```python
from build123d import *

# Parameters (mm, degrees)
BOSS_EXTRUDE1_DEPTH = 5.07492
SKETCH5_W           = 44.45
SKETCH5_H           = 127
BOSS_EXTRUDE2_DEPTH = 5.07492
SKETCH6_R           = 22.225
BOSS_EXTRUDE3_DEPTH = 5.07492
SKETCH2_3_R         = 6.35
CUT_EXTRUDE2_DEPTH  = 5.588
SKETCH8_W           = 2.728150378
SKETCH8_H           = 119.38
BOSS_EXTRUDE4_DEPTH = 5.07492
SKETCH9_R           = 3
CUT_EXTRUDE3_DEPTH  = 400.05
SKETCH10_R          = 2.54
SKETCH10_R_2        = 3.175
CUT_EXTRUDE4_DEPTH  = 6.35


with BuildPart() as part:
    # Sketch2 → Boss-Extrude1 (new body)
    with BuildSketch(Plane.XY):
        with BuildLine():
            Line((-143.383, -31.75), (-127.127, -31.75))
            ThreePointArc((-127.127, -31.75), (-123.317, -30.48), (-119.507, -31.75))
            Line((-119.507, -31.75), (119.253, -31.75))
            ThreePointArc((119.253, -31.75), (123.063, -30.48), (126.873, -31.75))
            Line((126.873, -31.75), (143.383, -31.75))
            Line((143.383, -31.75), (143.383, 95.25))
            Line((143.383, 95.25), (-143.383, 95.25))
            Line((-143.383, 95.25), (-143.383, -31.75))
        make_face()
    extrude(amount=-BOSS_EXTRUDE1_DEPTH)

    # Sketch5 → Boss-Extrude2 (add)
    with BuildSketch(Plane(origin=(0, 0, -5.07492), x_dir=(-1, 0, 0), z_dir=(0, 0, -1))):
        with Locations((-165.608, 31.75)):
            Rectangle(SKETCH5_W, SKETCH5_H)
    extrude(amount=-BOSS_EXTRUDE2_DEPTH)

    # Sketch6 → Boss-Extrude3 (add)
    with BuildSketch(Plane(origin=(0, 0, -5.07492), x_dir=(-1, 0, 0), z_dir=(0, 0, -1))):
        with Locations((-123.063, -36.83)):
            Circle(SKETCH6_R)
        with Locations((123.317, -36.83)):
            Circle(SKETCH6_R)
    extrude(amount=-BOSS_EXTRUDE3_DEPTH)

    # Sketch2<3> → Cut-Extrude2 (cut)
    with BuildSketch(Plane.XY):
        with Locations((-123.317, -36.83)):
            Circle(SKETCH2_3_R)
        with Locations((123.063, -36.83)):
            Circle(SKETCH2_3_R)
    extrude(amount=-CUT_EXTRUDE2_DEPTH, mode=Mode.SUBTRACT)

    # Sketch8 → Boss-Extrude4 (add)
    with BuildSketch(Plane(origin=(0, 0, -5.07492), x_dir=(-1, 0, 0), z_dir=(0, 0, -1))):
        with Locations((144.139824811, 35.56)):
            Rectangle(SKETCH8_W, SKETCH8_H)
    extrude(amount=-BOSS_EXTRUDE4_DEPTH)

    # Sketch9 → Cut-Extrude3 (cut)
    with BuildSketch(Plane(origin=(0, 0, -5.07492), x_dir=(-1, 0, 0), z_dir=(0, 0, -1))):
        with Locations((-123.063, 76.2)):
            Circle(SKETCH9_R)
        with Locations((123.317, 76.2)):
            Circle(SKETCH9_R)
    extrude(amount=-CUT_EXTRUDE3_DEPTH, mode=Mode.SUBTRACT)

    # Sketch10 → Cut-Extrude4 (cut)
    with BuildSketch(Plane(origin=(0, 0, -5.07492), x_dir=(-1, 0, 0), z_dir=(0, 0, -1))):
        with Locations((-22.0091, -6.35)):
            Circle(SKETCH10_R)
        with Locations((31.9659, -6.35)):
            Circle(SKETCH10_R)
        with Locations((14.745829779, -23.114)):
            Circle(SKETCH10_R_2)
    extrude(amount=-CUT_EXTRUDE4_DEPTH, mode=Mode.SUBTRACT)


solid = part.part
```
Could you check a few things on this model? Use its own coordinates, in mm. Round coordinates to 2 decimals unless told otherwise and drop trailing zeros. Loops run counter-clockwise (first coordinate to the right, second up) from the corner with the lowest first, then second, coordinate; pieces in that order, holes last. Notation, with made-up numbers: M -2.5,11 L 39.5,11 A11 ccw 39.5,23 Z; hole C -28,-22 d3. An arc over 180 degrees is marked long. Write item = value, one per line.
1. I need wall thicknesses on probe 1 along X at (y, z) = (-6.5, -3.3); probe 2 along X at (y, z) = (-23.5, -1.25); probe 3 along X at (y, z) = (-34.5, -0.65). Which ranges of each line are inside material? Lowest first, please.
Results below:
probe_1 = -145.5 to -34.5, -29.43 to 19.47, 24.54 to 187.83
probe_2 = -145.5 to -17.9, -11.59 to 187.83
probe_3 = -145.42 to -129.22, -117.41 to -101.21, 100.96 to 117.16, 128.97 to 145.17
2. I want a section at A-A, the plane y = 76.2. Write out the boundary of the cut face in (x, z).
Results below:
outline = M -145.5,-5.07 L -126.32,-5.07 L -126.32,0 L -145.5,0 Z; M -120.32,-5.07 L 120.06,-5.07 L 120.06,0 L -120.32,0 Z; M 126.06,-5.07 L 187.83,-5.07 L 187.83,0 L 126.06,0 Z
3. I want a section at D-D, the plane x = 159.5. Write out the boundary of the cut face in (y, z), and give its area (3 significant figures).
Results below:
outline = M -31.75,-5.07 L 95.25,-5.07 L 95.25,0 L -31.75,0 Z
area = 645 mm²
4. Thinking about a two-plate mould opening in Y: for faces 1 (the face through (23, 36, 0)), 2 (the face through (-126.18, 77.1, -2.57)), which applies, +Y half, -Y half, draft (parallel to the pull), parting line (faces both ways), or undercut?
Results below:
face_1 = draft
face_2 = undercut
5. I want a section at B-B, the plane y = -36.83. Write out the boundary of the cut face in (x, z).
Results below:
outline = M -145.54,-5.07 L -129.67,-5.07 L -129.67,0 L -145.54,0 Z; M -116.97,-5.07 L -101.09,-5.07 L -101.09,0 L -116.97,0 Z; M 100.84,-5.07 L 116.71,-5.07 L 116.71,0 L 100.84,0 Z; M 129.41,-5.07 L 145.29,-5.07 L 145.29,0 L 129.41,0 Z
6. Will these pins go through, and if not, where does the flat tip stop? P1, Ø1.5, axis at x = 79, y = 54.5, coming from the +Z side; P2, Ø3, axis at x = 15, z = -0.5, coming from the -Y side; P3, Ø5, axis at x = 123.063, y = 76.2, coming from the +Z side; P4, Ø2.5, axis at x = -144, z = -1.5, coming from the -Y side.
Results below:
P1 = 0
P2 = -31.75
P3 = through
P4 = -47.61
7. I want a section at C-C, the plane z = -3.45. Write out the boundary of the cut face in (x, y) (3 decimals).
Results below:
outline = M -145.504,-24.13 L -143.383,-24.13 L -143.383,-27.275 A22.225 ccw long -101.68,-31.75 L 101.426,-31.75 A22.225 ccw long 144.7,-31.75 L 187.833,-31.75 L 187.833,95.25 L -145.504,95.25 Z; hole C -123.317,-36.83 d12.7; hole C -123.317,76.2 d6; hole C -31.966,-6.35 d5.08; hole C -14.746,-23.114 d6.35; hole C 22.009,-6.35 d5.08; hole C 123.063,-36.83 d12.7; hole C 123.063,76.2 d6
